Autodesk Inventor part; units mm, degrees
ref_plane "YZ Plane" through (0, 0, 0) normal (1, 0, 0) x (0, 1, 0)
ref_plane "XZ Plane" through (0, 0, 0) normal (0, 1, 0) x (-1, 0, 0)
ref_plane "XY Plane" through (0, 0, 0) normal (0, 0, 1) x (1, 0, 0)
sketch "Sketch1" plane through (0, 0, 0) normal (0, 0, 1) x (1, 0, 0)
  line L0 (0, 0) -> (0, 56)
  line L1 (0, 56) -> (6, 56)
  line L2 (6, 56) -> (6, 6)
  line L3 (6, 6) -> (70, 6)
  line L4 (70, 6) -> (70, 0)
  line L5 (70, 0) -> (0, 0)
  dimension "d0" = 56
  dimension "d1" = 6
  dimension "d2" = 50
  dimension "d3" = 64
  dimension "d4" = 6
extrude "Extrusion1" add sketch "Sketch1" along normal blind 40
sketch "Sketch2" plane through (6, 6, 0) normal (0, 1, 0) x (1, 0, 0)
  line L0 (0, 0) -> (0, -40)
  circle A0 centre (53, -20) radius 6.35
  line L1 (64, 0) -> (0, 0)
  line L2 (64, -40) -> (0, -40)
  point P0 (-6, 0)
  dimension "d8" = 12.7
  dimension "d25" = 53
extrude "Extrusion2" cut sketch "Sketch2" against normal blind 40
sketch "Sketch3" plane through (6, 6, 0) normal (1, 0, 0) x (0, 0, -1)
  line L0 (0, 50) -> (-40, 50)
  line L1 (-29.3643, 50) -> (-9.3643, 50)
  line L2 (-9.3643, 50) -> (-9.3643, 15)
  line L3 (-9.3643, 15) -> (-29.3643, 15)
  line L4 (-29.3643, 15) -> (-29.3643, 50)
  point P0 (0, -6)
  dimension "d13" = 20
  dimension "d14" = 35
extrude "Extrusion3" cut sketch "Sketch3" against normal blind 10
sketch "Sketch4" plane through (6, 6, 0) normal (1, 0, 0) x (0, 0, -1)
  circle A0 centre (-35, 40) radius 3.25
  line L0 (-40, 0) -> (-40, 50)
  line L1 (-29.3643, 50) -> (-40, 50)
  point P0 (0, -6)
  dimension "d17" = 6.5
  dimension "d18" = 5
  dimension "d19" = 10
extrude "Extrusion4" cut sketch "Sketch4" against normal blind 10
pattern_linear "Rectangular Pattern1" count 2 spacing 30 along (0, 0, -1) of "Extrusion4"
properties part number "motor_angle"
Here's how the part is built. I have some questions about the finished solid (model axes, mm). A direction names the side the tool comes from. Give positions to 0.01 mm unless a question says otherwise; leave off trailing zeros. Order: outer loops, then holes, each group sorted by start corner. A loop starts at its lowest first (then second) coordinate and runs counter-clockwise, first axis right, second up. Notation, with made-up numbers: (50, 65.5) -> (100, 65.5) arc R18 ccw to (100, 92.5) -> close; hole circle Ø5 at (48.5, 7.5). An arc over 180 degrees is marked (long way). Use CSV: the item, a comma, the result in double quotes. Start each with the question number.
Item 1: If I drill on probe 1 along X at (y, z) = (1, 20); probe 2 along Z at (x, y) = (59, 1.45); probe 3 along Y at (x, z) = (3.5, 35), over which ranges is the centre line in solid material (lowest first)? Write a range as [from, to].
Item 2: Suppose I cut it at C-C (y = 52). List the corners of the cut face in (x, z) for me, and give its area (3 significant figures).
Item 3: Thinking about a two-plate mould opening in Z: for faces 1 (the cylindrical face through (3.042, 42.827, 5.705)), 2 (the flat face through (22, 5, 40)), 3 (the flat face through (6, 20, 20)), which applies, pulls with the +Z half, pulls with the -Z half, needs draft (parallel to the pull), parting line crosses it, or undercut?
Item 4: Suppose I cut it at A-A (z = 35). List the corners of the cut face in (x, y) for me.
Item 5: Suppose I cut it at D-D (z = 20). List the corners of the cut face in (x, y) for me, and give its area (3 significant figures).
Item 6: I'm going to push flat-ended pins straight in: P1, Ø8.5, axis at y = 46, z = 5, coming from the +X side; P2, Ø3, axis at x = 30, z = 11, coming from the +Y side; P3, Ø6.5, axis at x = 2, z = 22, coming from the +Y side. Where does each tip first touch, or does it pass through?
Item 7: On a 3-axis mill with a long thin cutter (end or side, diameter ignored), from which of +Z, -Z, +X, -X, +Y, -Y can I reach the whole of each face in a straight line? I mean faces 4 (the flat face through (3, 39, 9.364)), 5 (the flat face through (38, 6, 20)), 6 (the cylindrical face through (53.96, 3.04, 23.86)). Say none if no direction works.
Item 8: Suppose I cut it at B-B (y = 46). List the corners of the cut face in (x, z) for me, and give its area (3 significant figures).
Answer block:
1,probe 1,"x = [0, 52.65], [65.35, 70]"
1,probe 2,"z = [0, 13.65], [26.35, 40]"
1,probe 3,"y = [0, 42.75], [49.25, 56]"
2,outline,"(0, 0) -> (6, 0) -> (6, 9.36) -> (0, 9.36) -> close; (0, 29.36) -> (6, 29.36) -> (6, 40) -> (0, 40) -> close"
2,area,"120 mm^2"
3,face 1,"undercut"
3,face 2,"pulls with the +Z half"
3,face 3,"needs draft"
4,outline,"(0, 0) -> (70, 0) -> (70, 6) -> (6, 6) -> (6, 42.75) -> (0, 42.75) -> close; (0, 49.25) -> (6, 49.25) -> (6, 56) -> (0, 56) -> close"
5,outline,"(0, 0) -> (52.65, 0) -> (52.65, 6) -> (6, 6) -> (6, 21) -> (0, 21) -> close; (65.35, 0) -> (70, 0) -> (70, 6) -> (65.35, 6) -> close"
5,area,"434 mm^2"
6,P1,"stops at x = 6"
6,P2,"stops at y = 6"
6,P3,"stops at y = 21"
7,face 4,"+X, -X, +Y"
7,face 5,"+Z, -Z, +X, +Y"
7,face 6,"+Y, -Y"
8,outline,"(0, 0) -> (6, 0) -> (6, 1.75) -> (0, 1.75) -> close; (0, 8.25) -> (6, 8.25) -> (6, 9.36) -> (0, 9.36) -> close; (0, 29.36) -> (6, 29.36) -> (6, 31.75) -> (0, 31.75) -> close; (0, 38.25) -> (6, 38.25) -> (6, 40) -> (0, 40) -> close"
8,area,"42.0 mm^2"
